from build123d import *

# Parameters (mm, degrees)
SKETCH2_W               = 50.8
SKETCH2_H               = 50.8
BASE_FLANGE1_DEPTH      = 2.54
FILLET1_R               = 9.017
SKETCH9_R               = 9.525
BOSS_EXTRUDE1_DEPTH     = 2.54
SKETCH10_R              = 8.255
CUT_EXTRUDE1_DEPTH      = 2.286
SKETCH11_R              = 6.35
CUT_EXTRUDE2_DEPTH      = 37.029521729
SKETCH12_R              = 3.175
CUT_EXTRUDE4_DEPTH      = 37.278456417
MIRROR2_COPY_1_SKETCH_R = 3.175
MIRROR2_COPY_1_DEPTH    = 37.278456417
CHAMFER1_SIZE           = 1.27


# Sheet-metal steps are written as plain solids
with BuildPart() as part:
    # Sketch2 → Base-Flange1 (new body)
    with BuildSketch(Plane(origin=(0, 0, 0), x_dir=(1, 0, 0), z_dir=(0, 1, 0))):
        Rectangle(SKETCH2_W, SKETCH2_H)
    extrude(amount=-BASE_FLANGE1_DEPTH)

    # Fillet1
    fillet1_edges = [part.edges().sort_by_distance(p)[0] for p in [
        (25.4, -1.27, 25.4),
        (-25.4, -1.27, 25.4),
        (-25.4, -1.27, -25.4),
        (25.4, -1.27, -25.4),
    ]]
    fillet(fillet1_edges, radius=FILLET1_R)

    # Sketch9 → Boss-Extrude1 (add)
    with BuildSketch(Plane(origin=(0, 0, 0), x_dir=(1, 0, 0), z_dir=(0, 1, 0))):
        with Locations(Location((0, 0, 0), (0, 0, 270))):
            Circle(SKETCH9_R)
    extrude(amount=BOSS_EXTRUDE1_DEPTH)

    # Sketch10 → Cut-Extrude1 (cut)
    with BuildSketch(Plane.XZ.offset(2.54)):
        with Locations(Location((0, 0, 0), (0, 0, 270))):
            Circle(SKETCH10_R)
    extrude(amount=-CUT_EXTRUDE1_DEPTH, mode=Mode.SUBTRACT)

    # Sketch11 → Cut-Extrude2 (cut, through all)
    with BuildSketch(Plane.XZ.offset(0.254)):
        with Locations(Location((0, 0, 0), (0, 0, 270))):
            Circle(SKETCH11_R)
    extrude(amount=-CUT_EXTRUDE2_DEPTH, mode=Mode.SUBTRACT)

    # Sketch12 → Cut-Extrude4 (cut, through all)
    with BuildSketch(Plane.XZ.offset(2.54)):
        with Locations(Location((-16.383, -16.383, 0), (0, 0, 270))):
            Circle(SKETCH12_R)
    cut_extrude4 = extrude(amount=-CUT_EXTRUDE4_DEPTH, mode=Mode.SUBTRACT)

    # Mirror1: Cut-Extrude4 across plane
    add(cut_extrude4.mirror(Plane(origin=(0, 0, 0), x_dir=(0, 0, 1), z_dir=(1, 0, 0))), mode=Mode.SUBTRACT)

    # Mirror2: Cut-Extrude4 across plane
    add(cut_extrude4.mirror(Plane.XY), mode=Mode.SUBTRACT)

    # Mirror2 copy 1 sketch → Mirror2 copy 1 (cut, through all)
    with BuildSketch(Plane(origin=(0, -2.54, 0), x_dir=(-1, 0, 0), z_dir=(0, -1, 0))):
        with Locations(Location((-16.383, -16.383, 0), (0, 0, 270))):
            Circle(MIRROR2_COPY_1_SKETCH_R)
    extrude(amount=-MIRROR2_COPY_1_DEPTH, mode=Mode.SUBTRACT)

    # Chamfer1
    chamfer1_edges = [part.edges().sort_by_distance(p)[0] for p in [
        (-16.383, 0, -13.208),
        (16.383, 0, -13.208),
        (16.383, 0, 13.208),
        (-16.383, 0, 13.208),
    ]]
    chamfer(chamfer1_edges, length=CHAMFER1_SIZE)


solid = part.part
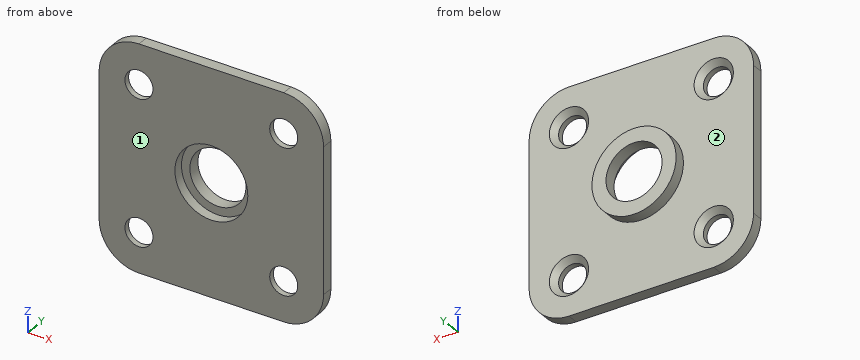
Geometry: final body of the model. Coordinates: model frame, mm. Face numbers are marked on the shaded views. A direction names the side the tool comes from. Round coordinates to 2 decimals unless told otherwise and drop trailing zeros. Loops run counter-clockwise (first coordinate to the right, second up) from the corner with the lowest first, then second, coordinate; pieces in that order, holes last.
Q1. Section D-D on x = 7. Return loops of the section in (y, z).
Q2. Pin query (flat end, axial travel): P1, Ø8, axis at x = -8, z = 17, coming from the +Y side; P2, Ø4, axis at x = 16, z = 14.5, coming from the +Y side; P3, Ø4, axis at x = 16.383, z = -16.383, coming from the -Y side; P4, Ø4, axis at x = 0.5, z = -5, coming from the -Y side. Return the tip coordinate at first contact, or that it passes through.
Q3. Section A-A on z = 0. Return loops of the section in (x, y) (3 decimals).
Q4. Access query for the marked faces 1 and 2. Directions: +Z, -Z, +X, -X, +Y, -Y. A direction counts if a zero-diameter tool reaches every point of the face in a straight line with its end or side. Return the directions, or none.
Q5. Material intervals for L1, parallel to Z at x = -0.5, y = -1.8; L2, parallel to Y at x = -23, z = 6; L3, parallel to Z at x = 13.5, y = -1.35, sorted ascending.
Q6. Section C-C on y = 0.65. Return loops of the section in (x, z) (3 decimals).
Q7. Section B-B on x = 0. Return loops of the section in (y, z) (3 decimals), plus the area to 3 significant figures.
Evaluation:
1. outline: (-2.54, -25.4) - (0, -25.4) - (0, -6.46) - (2.54, -6.46) - (2.54, 6.46) - (0, 6.46) - (0, 25.4) - (-2.54, 25.4) - (-2.54, 4.38) - (-0.25, 4.38) - (-0.25, -4.38) - (-2.54, -4.38) - close
2. P1: stops at y = 0
2. P2: stops at y = -0.52
2. P3: passes through
2. P4: stops at y = -0.25
3. outline: (-25.4, -2.54) - (-8.255, -2.54) - (-8.255, -0.254) - (-6.35, -0.254) - (-6.35, 2.54) - (-9.525, 2.54) - (-9.525, 0) - (-25.4, 0) - close; (6.35, -0.254) - (8.255, -0.254) - (8.255, -2.54) - (25.4, -2.54) - (25.4, 0) - (9.525, 0) - (9.525, 2.54) - (6.35, 2.54) - close
4. face 1: +Z, -Z, +X, -X, -Y
4. face 2: +Y
5. L1: z = -25.4 to -8.24, 8.24 to 25.4
5. L2: y = -2.54 to 0
5. L3: z = -25.4 to -17.71, -15.05 to 15.05, 17.71 to 25.4
6. outline: circle Ø19.05 at (0, 0); hole circle Ø12.7 at (0, 0)
7. outline: (-2.54, -25.4) - (0, -25.4) - (0, -9.525) - (2.54, -9.525) - (2.54, -6.35) - (-0.254, -6.35) - (-0.254, -8.255) - (-2.54, -8.255) - close; (-2.54, 8.255) - (-0.254, 8.255) - (-0.254, 6.35) - (2.54, 6.35) - (2.54, 9.525) - (0, 9.525) - (0, 25.4) - (-2.54, 25.4) - close
7. area: 104 mm2
